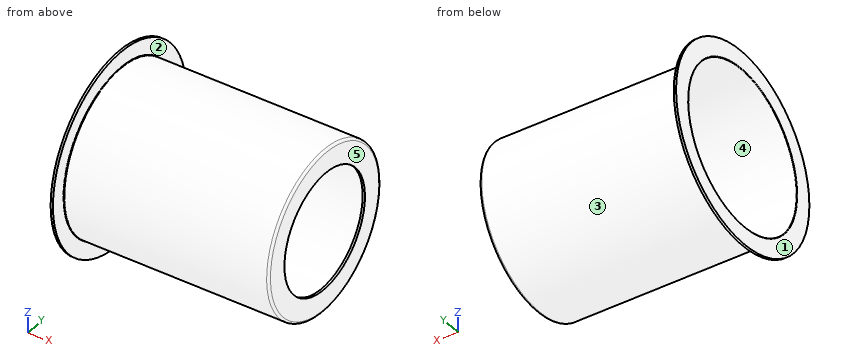
from build123d import *


with BuildPart() as f1:
    # F0 (on Front) → F1 (revolve)
    with BuildSketch(Plane.XZ):
        with BuildLine():
            Line((-5, 179.7), (-449, 179.7))
            ThreePointArc((-449, 179.7), (-449.707107, 179.992893), (-450, 180.7))
            Line((-450, 180.7), (-450, 214.7))
            Line((-450, 214.7), (-455, 214.7))
            Line((-455, 214.7), (-455, 176))
            ThreePointArc((-455, 176), (-454.619239, 175.080761), (-453.7, 174.7))
            Line((-453.7, 174.7), (-9.7, 174.7))
            ThreePointArc((-9.7, 174.7), (-6.376598, 173.323402), (-5, 170))
            Line((-5, 170), (-5, 129.7))
            Line((-5, 129.7), (0, 129.7))
            Line((0, 129.7), (0, 174.7))
            ThreePointArc((0, 174.7), (-1.464466, 178.235534), (-5, 179.7))
        make_face()
    revolve(axis=Axis((9.014154, 0, 0), (1, 0, 0)))


solid = f1.part
CAD build for the part. Positions are in the model's coordinates, mm. Face numbers are marked on the shaded views. A direction names the side the tool comes from. Round coordinates to 2 decimals unless told otherwise and drop trailing zeros. Loops run counter-clockwise (first coordinate to the right, second up) from the corner with the lowest first, then second, coordinate; pieces in that order, holes last. Notation, with made-up numbers: M 63,-29.75 L 121,-29.75 A4 cw 121,-24.75 Z; hole C -28.75,-9 d1. An arc over 180 degrees is marked long. One line per question, with ' | ' between items. Start each with the question number.
Item 1: Cut at A-A, the plane z = 0. Write the cut outline in (x, y), plus the area to 3 significant figures.
Item 2: Wall check: line 1 (Z direction, x = -203, y = 0); line 2 (Y direction, x = -152, z = 1.5); line 3 (Y direction, x = -301, z = 6). Give the ranges that are in metal, low to high.
Item 3: Cut at C-C, the plane x = -246. Write the cut outline in (y, z), plus the area to 3 significant figures.
Item 4: Pin check, flat tips, straight feed: pin 1 Ø5 at (x, z) = (-350.5, 78) entering from +Y; pin 2 Ø8 at (x, z) = (-324.5, -109) entering from +Y; pin 3 Ø2 at (x, z) = (-390.5, 3) entering from +Y. Stop position of each tip, or through.
Item 5: Which spindle directions (+Z, -Z, +X, -X, +Y, -Y) get a long thin tool onto all of the face, cutting with end or side? Do the marked faces 1 and 2. Say none if no direction does.
Item 6: Two-plate mould, pull along Z, no slides. Class the marked faces 3, 4 and 5: pulls with the +Z half, pulls with the -Z half, needs draft (parallel to the pull), parting line crosses it, or undercut.
Responses:
1) outline: M -455,-214.7 L -450,-214.7 L -450,-180.7 A1 cw -449,-179.7 L -5,-179.7 A5 ccw 0,-174.7 L 0,-129.7 L -5,-129.7 L -5,-170 A4.7 cw -9.7,-174.7 L -453.7,-174.7 A1.3 ccw -455,-176 Z; M -455,176 A1.3 ccw -453.7,174.7 L -9.7,174.7 A4.7 cw -5,170 L -5,129.7 L 0,129.7 L 0,174.7 A5 ccw -5,179.7 L -449,179.7 A1 cw -450,180.7 L -450,214.7 L -455,214.7 Z | area: 5,350 mm²
2) line 1: z = -179.7 to -174.7, 174.7 to 179.7 | line 2: y = -179.69 to -174.69, 174.69 to 179.69 | line 3: y = -179.6 to -174.6, 174.6 to 179.6
3) outline: C 0,0 d359.4; hole C 0,0 d349.4 | area: 5,570 mm²
4) pin 1: stops at y = 163.07 | pin 2: stops at y = 145.83 | pin 3: stops at y = 179.69
5) face 1: +Z, -Z, -X, +Y, -Y | face 2: +X
6) face 3: parting line crosses it | face 4: undercut | face 5: needs draft
